Source: CAD feature listing. Evaluate the final solid. Frame: model axes, mm. Coordinates: 2 decimals unless noted, no trailing zeros. Order: outer loops, then holes, each group sorted by start corner. A loop starts at its lowest first (then second) coordinate and runs counter-clockwise, first axis right, second up. Notation, with made-up numbers: (50.5, 46) - (103.5, 46) arc R32 cw to (103.5, 72) - close; hole circle Ø3 at (20.5, -0.5). An arc over 180 degrees is marked (long way). One line per question, with ' | ' between items. Start each with the question number.
(1) Contact query for flat-ended pins moving along their axis: P1, Ø2, axis at y = -10.5, z = 1, coming from the -X side; P2, Ø6, axis at x = 8, y = 2, coming from the +Z side; P3, Ø1.1, axis at x = 0, z = 5.5, coming from the +Y side (3 decimals). Output: stop coordinate, or through.
(2) Line query: line 1 along Z through (x, y) = (-9, 4); line 2 along X through (y, z) = (2.5, 5.75); line 3 along Y through (x, z) = (6, 4.5). Output: solid intervals per line, ascending.
(3) Section B-B (z = 4.25). Return the cut outline in (x, y) (3 decimals).
(4) Section A-A (x = 0). Return the cut outline in (y, z), then the cut area to 4 significant figures.
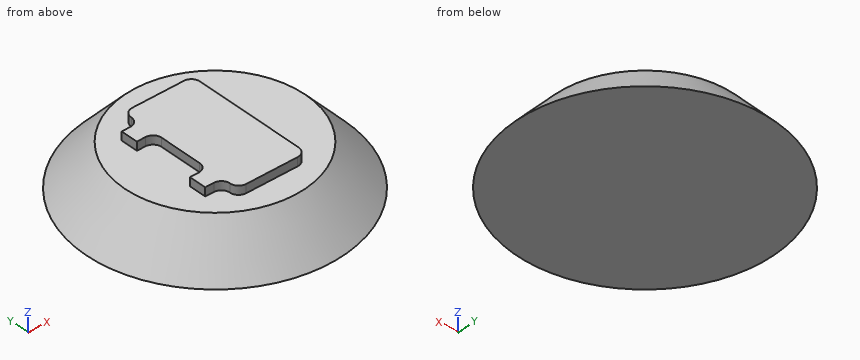
from build123d import *

# Parameters (mm, degrees)
F0_R     = 15
F2_R     = 10.5
F5_DEPTH = 1
F6_R     = 0.99999


# Not quite as in the source:
# - a fillet or chamfer is up to 0.001 mm smaller than in the source, because OpenCascade refuses the exact size


with BuildPart() as f3:
    # F0 (on Top) → F3 section 0
    with BuildSketch(Plane.XY):
        Circle(F0_R)
    # F2 (on offset) → F3 section 1
    with BuildSketch(Plane.XY.offset(5)):
        Circle(F2_R)
    loft()

    # F4 (on face) → F5 (join)
    with BuildSketch(Plane.XY.offset(5)):
        Polygon((-4, -5.5), (-4, -7.5), (4, -7.5), (4, 7.5), (-4, 7.5), (-4, 5.5), (-6, 5.5), (-6, 3.5), (-4, 3.5), (-4, -3.5), (-6, -3.5), (-6, -5.5), align=None)
    extrude(amount=F5_DEPTH)

    # F6 (radius 1 in the source; OpenCascade refuses exactly that, so slightly less here)
    f6_edges = [f3.edges().sort_by_distance(p)[0] for p in [
        (-4, -7.5, 5.5),
        (4, -7.5, 5.5),
        (4, 7.5, 5.5),
        (-4, 7.5, 5.5),
        (-4, -5.5, 5.5),
        (-4, 3.5, 5.5),
        (-4, -3.5, 5.5),
        (-4, 5.5, 5.5),
    ]]
    fillet(f6_edges, radius=F6_R)


solid = f3.part
Response values:
1) P1: stops at x = -11.03 | P2: stops at z = 5 | P3: stops at y = 10.545
2) line 1: z = 0 to 5 | line 2: x = -4 to 4 | line 3: y = -9.16 to 9.16
3) outline: circle Ø22.35 at (0, 0)
4) outline: (-15, 0) - (15, 0) - (10.5, 5) - (7.5, 5) - (7.5, 6) - (-7.5, 6) - (-7.5, 5) - (-10.5, 5) - close | area: 142.5 mm²
